Design review of the part shown in the three views and the two pictorial views. Dimensions are in mm from the part's minimum x, y and z. A direction names the side the tool comes from. Round coordinates to 2 decimals unless told otherwise and drop trailing zeros. Loops run counter-clockwise (first coordinate to the right, second up) from the corner with the lowest first, then second, coordinate; pieces in that order, holes last.
1. Consider section B-B on y = 40. State the section outline as (x, z) points.
2. Draft analysis for pull direction X (two halves, no side actions). For the marked faces 6, 7 and 8, state which applies: released by +X, released by -X, zero draft, split by the parting line, or undercut.
3. To check wall thickness, follow line 1 along X through (y, z) = (92.7, 40); line 2 along Z through (x, y) = (37, 93) (1 decimal); line 3 along Y through (x, z) = (27, 39) (1 decimal). State the ranges of each line that lie inside material, in increasing order.
4. Tool access review of the marked faces 1, 2, 3, 4 and 5: name each direction out of +Z, -Z, +X, -X, +Y, -Y from which nothing blocks a thin tool from reaching the whole face with its end or side.
5. Consider section A-A on z = 24.5. State the section outline as (x, y) points.
6. Consider section D-D on y = 92.7. State the section outline as (x, z) points (1 decimal).
7. Clearance check with flat-ended pins moving along their axes: pin 1 Ø6 at (x, y) = (55.5, 64.5) entering from -Z; pin 2 Ø1.5 at (y, z) = (56, 31.5) entering from -X; pin 3 Ø9 at (x, y) = (52.7, 92.7) entering from +Z (3 decimals); pin 4 Ø11 at (x, y) = (52.7, 92.7) entering from -Z (3 decimals). State where each tip first meets the part, or that it passes through.
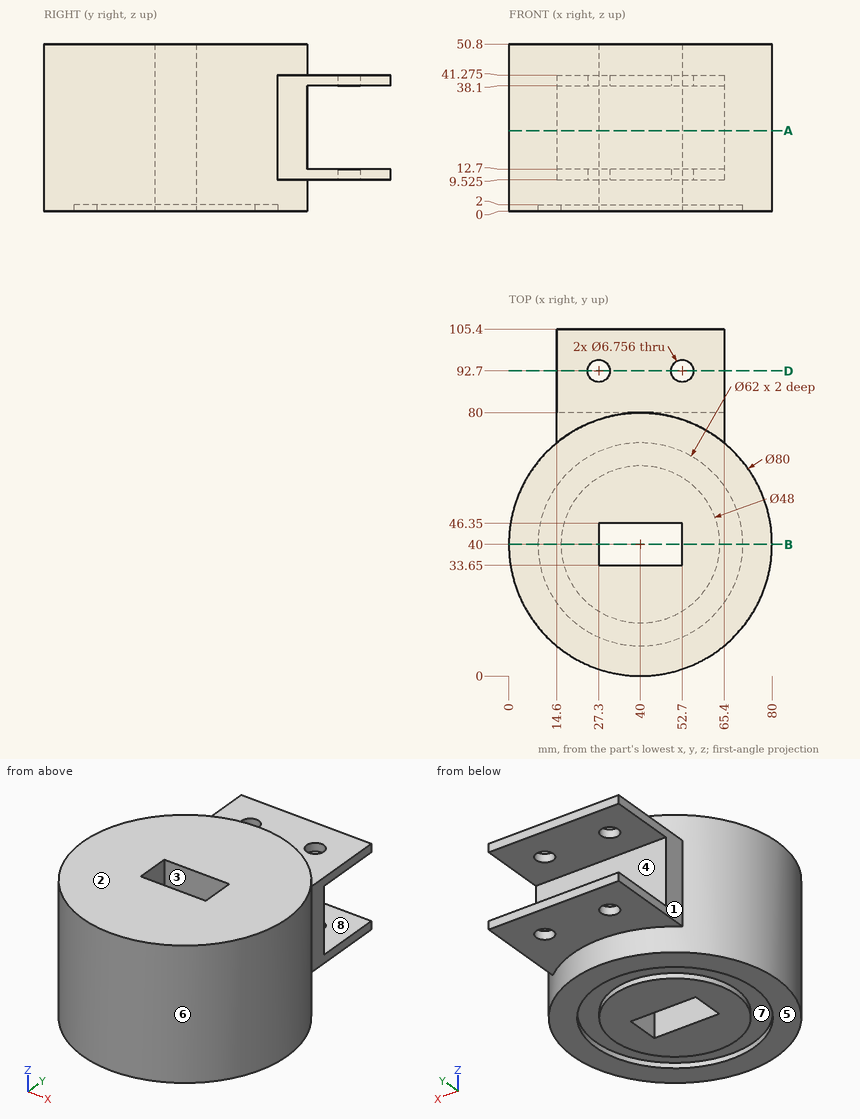
Resolved:
1. outline: (0, 0) - (9, 0) - (9, 2) - (16, 2) - (16, 0) - (27.3, 0) - (27.3, 50.8) - (0, 50.8) - close; (52.7, 0) - (64, 0) - (64, 2) - (71, 2) - (71, 0) - (80, 0) - (80, 50.8) - (52.7, 50.8) - close
2. face 6: split by the parting line
2. face 7: undercut
2. face 8: zero draft
3. line 1: x = 14.6 to 23.92, 30.68 to 49.32, 56.08 to 65.4
3. line 2: z = 9.5 to 12.7, 38.1 to 41.3
3. line 3: y = 2.2 to 89.3, 96.1 to 105.4
4. face 1: +Z, -Z, -X, +Y
4. face 2: +Z, +X, -X, +Y, -Y
4. face 3: +Z, -Z
4. face 4: +X, -X, +Y
4. face 5: -Z, +X, -X, +Y, -Y
5. outline: (14.6, 70.9) arc R40 ccw (long way) to (65.4, 70.9) - (65.4, 80) - (14.6, 80) - close; hole (27.3, 33.65) - (52.7, 33.65) - (52.7, 46.35) - (27.3, 46.35) - close
6. outline: (14.6, 9.5) - (23.9, 9.5) - (23.9, 12.7) - (14.6, 12.7) - close; (14.6, 38.1) - (23.9, 38.1) - (23.9, 41.3) - (14.6, 41.3) - close; (30.7, 9.5) - (49.3, 9.5) - (49.3, 12.7) - (30.7, 12.7) - close; (30.7, 38.1) - (49.3, 38.1) - (49.3, 41.3) - (30.7, 41.3) - close; (56.1, 9.5) - (65.4, 9.5) - (65.4, 12.7) - (56.1, 12.7) - close; (56.1, 38.1) - (65.4, 38.1) - (65.4, 41.3) - (56.1, 41.3) - close
7. pin 1: stops at z = 0
7. pin 2: stops at x = 3.02
7. pin 3: stops at z = 41.275
7. pin 4: stops at z = 9.525
